from build123d import *

# Parameters (mm, degrees)
BOSS_EXTRUDE1_DEPTH              = 6.35
SKETCH2_W                        = 203.2
SKETCH2_H                        = 6.35
BOSS_EXTRUDE2_DEPTH              = 330.2
BOSS_EXTRUDE3_DEPTH              = 6.35
F_17_64_0_26563_DIAMETER_HOLE1_D = 6.747002
CONVERT_SOLID1_START             = -101.6
CONVERT_SOLID1_DEPTH             = 203.2
CONVERT_SOLID1_2_DEPTH           = 203.2
F_5_32_0_15625_DIAMETER_HOLE1_D  = 3.96875
FILLET1_R                        = 6.35
FILLET2_R                        = 6.35


# Read off the part's stored shape, not the designer's step: Convert-Solid1
with BuildPart() as part:
    # Sketch1 → Boss-Extrude1 (new body)
    with BuildSketch(Plane(origin=(0, 0, 0), x_dir=(1, 0, 0), z_dir=(0, 1, 0))):
        Polygon((-215.9, 107.95), (-215.9, 63.5), (-101.6, 63.5), (-101.6, 50.8), (-57.15, 50.8), (-57.15, 38.1), (-101.6, 38.1), (-101.6, 0), (101.6, 0), (101.6, 38.1), (57.15, 38.1), (57.15, 50.8), (101.6, 50.8), (101.6, 63.5), (215.9, 63.5), (215.9, 107.95), align=None)
    extrude(amount=BOSS_EXTRUDE1_DEPTH)

    # Sketch2 → Boss-Extrude2 (add)
    with BuildSketch(Plane.XZ):
        with Locations((0, -3.175)):
            Rectangle(SKETCH2_W, SKETCH2_H)
    extrude(amount=BOSS_EXTRUDE2_DEPTH)

    # Sketch3 → Boss-Extrude3 (add)
    with BuildSketch(Plane.XZ.offset(330.2)):
        Polygon((-215.9, -107.95), (215.9, -107.95), (215.9, -63.5), (101.6, -63.5), (101.6, -50.8), (57.15, -50.8), (57.15, -38.1), (101.6, -38.1), (101.6, 0), (-101.6, 0), (-101.6, -38.1), (-57.15, -38.1), (-57.15, -50.8), (-101.6, -50.8), (-101.6, -63.5), (-215.9, -63.5), align=None)
    extrude(amount=BOSS_EXTRUDE3_DEPTH)

    # 17/64 (0.26563) Diameter Hole1 (through all)
    with Locations(Plane(origin=(0, 6.35, 0), x_dir=(1, 0, 0), z_dir=(0, 1, 0))):
        with Locations((-193.675, 82.55), (193.675, 82.55)):
            Hole(F_17_64_0_26563_DIAMETER_HOLE1_D / 2)

    # Convert-Solid1 outline → Convert-Solid1 (cut)
    with BuildSketch(Plane.YZ.offset(CONVERT_SOLID1_START)):
        with BuildLine():
            Line((6.35, 0), (-6.35, 0))
            ThreePointArc((-6.35, 0), (2.630256121, -3.719743879), (6.35, -12.7))
            Line((6.35, -12.7), (6.35, 0))
        make_face()
        with BuildLine():
            ThreePointArc((-336.55, -12.7), (-332.830256121, -3.719743879), (-323.85, 0))
            Line((-323.85, 0), (-336.55, 0))
            Line((-336.55, 0), (-336.55, -12.7))
        make_face()
    extrude(amount=CONVERT_SOLID1_DEPTH, mode=Mode.SUBTRACT)

    # Convert-Solid1 2 outline → Convert-Solid1 2 (add)
    with BuildSketch(Plane.YZ.offset(CONVERT_SOLID1_START)):
        with BuildLine():
            Line((0, -6.35), (-6.35, -6.35))
            ThreePointArc((-6.35, -6.35), (-1.859871939, -8.209871939), (0, -12.7))
            Line((0, -12.7), (0, -6.35))
        make_face()
        with BuildLine():
            ThreePointArc((-330.2, -12.7), (-328.340128061, -8.209871939), (-323.85, -6.35))
            Line((-323.85, -6.35), (-330.2, -6.35))
            Line((-330.2, -6.35), (-330.2, -12.7))
        make_face()
    extrude(amount=CONVERT_SOLID1_2_DEPTH)

    # 5/32 (0.15625) Diameter Hole1 (through all)
    with Locations(Plane(origin=(-44.7675, 6.35, -80.01), x_dir=(0, 0, 1), z_dir=(0, 1, 0))):
        with Locations((0, 0), (0, 17.78), (0, 71.755), (0, 89.535)):
            Hole(F_5_32_0_15625_DIAMETER_HOLE1_D / 2)

    # Fillet1
    fillet1_edges = [part.edges().sort_by_distance(p)[0] for p in [
        (57.15, -333.375, -38.1),
        (57.15, -333.375, -50.8),
        (57.15, 3.175, -38.1),
        (57.15, 3.175, -50.8),
        (-57.15, -333.375, -50.8),
        (-57.15, 3.175, -38.1),
        (-57.15, -333.375, -38.1),
        (-57.15, 3.175, -50.8),
    ]]
    fillet(fillet1_edges, radius=FILLET1_R - 0.0001)  # a hair under: the kernel refuses the full size

    # Fillet2
    fillet2_edges = [part.edges().sort_by_distance(p)[0] for p in [
        (101.6, 3.175, -63.5),
        (-101.6, 3.175, -63.5),
        (-101.6, -333.375, -63.5),
        (101.6, -333.375, -63.5),
    ]]
    fillet(fillet2_edges, radius=FILLET2_R)


solid = part.part
Input: part model. Units: mm. Frame: model coordinates. A direction names the side the tool comes from. Give positions to 0.01 mm unless a question says otherwise; leave off trailing zeros. Write each loop counter-clockwise with the first axis right and the second up, starting at its lowest first coordinate (ties: lowest second). Pieces come first, ordered by that corner, then holes. Notation, with made-up numbers: (-15, 24.25) -> (-2, 24.25) arc R28 cw to (-2, 58.25) -> close; hole circle Ø6 at (42.25, 72). An arc over 180 degrees is marked (long way). Use one line per item in the form item = value. Start each with the question number.
1) Section query A-A on x = -91. Return the cut outline in (y, z), then the cut area to 3 significant figures.
2) Section query B-B on z = -26. Return the cut outline in (x, y).
3) Draft query along Y for faces 1 (the flat face through (101.6, -191, -5)), 2 (the flat face through (-3, -330.2, -70)), 3 (the cylindrical face through (-1.42, 2.53, -3.62)), 4 (the flat face through (-3, 0, -72)). Return one class per face: pulls with the +Y half, pulls with the -Y half, needs draft (parallel to the pull), parting line crosses it, or undercut.
4) Section query D-D on y = -187. Return the cut outline in (x, z).
5) Ray query, probe 1 along Y at (x, z) = (-14, -52); probe 2 along X at (y, z) = (2.5, -82.55); probe 3 along Z at (x, y) = (52.5, -175). Return the intervals inside material, ascending. Write a range as from..to.
6) Set-up query: faces 5 (the flat face through (-101.6, -191, -5)), 6 (the flat face through (1, -163, 0)), 7 (the flat face through (-1, -163, -6.35)). Return all of +Z, -Z, +X, -X, +Y, -Y with unobstructed straight access to the full face (end or side cutting, diameter ignored); none if empty.
7) Pin query (flat end, axial travel): pin 1 (2.5 mm diameter, centred on x = -44.77, z = -80.01, fed in from +Y); pin 2 (5 mm diameter, centred on x = 90, y = -334, fed in from +Z); pin 3 (2 mm diameter, centred on x = -88.5, z = -38.5, fed in from +Y); pin 4 (3 mm diameter, centred on y = 3, z = -54, fed in from -X). Return the tip coordinate at first contact, or that it passes through.
8) Section query C-C on x = 150.5. Return the cut outline in (y, z).
Outcome:
q1.outline = (-336.55, -107.95) -> (-330.2, -107.95) -> (-330.2, -50.8) -> (-336.55, -50.8) -> close; (-336.55, -38.1) -> (-330.2, -38.1) -> (-330.2, -12.7) arc R6.35 cw to (-323.85, -6.35) -> (-6.35, -6.35) arc R6.35 cw to (0, -12.7) -> (0, -38.1) -> (6.35, -38.1) -> (6.35, -12.7) arc R12.7 ccw to (-6.35, 0) -> (-323.85, 0) arc R12.7 ccw to (-336.55, -12.7) -> close; (0, -107.95) -> (6.35, -107.95) -> (6.35, -50.8) -> (0, -50.8) -> close
q1.area = 3,250 mm^2
q2.outline = (-101.6, -336.55) -> (101.6, -336.55) -> (101.6, -330.2) -> (-101.6, -330.2) -> close; (-101.6, 0) -> (101.6, 0) -> (101.6, 6.35) -> (-101.6, 6.35) -> close
q3.face_1 = needs draft
q3.face_2 = undercut
q3.face_3 = pulls with the +Y half
q3.face_4 = undercut
q4.outline = (-101.6, -6.35) -> (101.6, -6.35) -> (101.6, 0) -> (-101.6, 0) -> close
q5.probe_1 = -336.55..-330.2, 0..6.35
q5.probe_2 = -215.9..-197.05, -190.3..190.3, 197.05..215.9
q5.probe_3 = -6.35..0
q6.face_5 = +Z, -X, +Y, -Y
q6.face_6 = +Z, +X, -X, +Y, -Y
q6.face_7 = -Z, +X, -X
q7.pin_1 = through
q7.pin_2 = -2.56
q7.pin_3 = 6.35
q7.pin_4 = -101.6
q8.outline = (-336.55, -107.95) -> (-330.2, -107.95) -> (-330.2, -63.5) -> (-336.55, -63.5) -> close; (0, -107.95) -> (6.35, -107.95) -> (6.35, -63.5) -> (0, -63.5) -> close
